Design review of the part built by this model. Coordinates are the model's own, in mm. A direction names the side the tool comes from. Coordinates: 2 decimals unless noted, no trailing zeros. Loops run counter-clockwise (first coordinate to the right, second up) from the corner with the lowest first, then second, coordinate; pieces in that order, holes last. Notation, with made-up numbers: (88.5, 64.5) -> (146.5, 64.5) arc R16 cw to (146.5, 95.5) -> close; hole circle Ø5 at (69, -28). An arc over 180 degrees is marked (long way). Answer as a JSON object with one key per item and string values.
```python
from build123d import *
from OCP.BRepFilletAPI import BRepFilletAPI_MakeChamfer

# Parameters (mm, degrees)
SKETCH_1_W          = 50
SKETCH_1_H          = 50
EXTRUDE_1_DEPTH     = 5
SKETCH_5_R          = 8
EXTRUDE_3_DEPTH     = 30
SKETCH_6_R          = 5.4
CUT_EXTRUDE_2_DEPTH = 50.749371855
FILLET_3_R          = 2
FILLET_2_SIZE       = 15
FILLET_2_SIZE_2     = 10
CHAMFER_1_SIZE      = 6
CHAMFER_1_SIZE2     = 2.797845949


with BuildPart() as part:
    # Эскиз1 → Бобышка-Вытянуть1 (new body)
    with BuildSketch(Plane(origin=(0, 0, 0), x_dir=(1, 0, 0), z_dir=(0, 1, 0))):
        Rectangle(SKETCH_1_W, SKETCH_1_H)
    extrude(amount=EXTRUDE_1_DEPTH)

    # Эскиз5 → Бобышка-Вытянуть3 (add)
    with BuildSketch(Plane(origin=(0, 5, 0), x_dir=(1, 0, 0), z_dir=(0, 1, 0))):
        with Locations(Location((0, 0, 0), (0, 0, 270))):
            Circle(SKETCH_5_R)
    extrude(amount=EXTRUDE_3_DEPTH)

    # Эскиз6 → Вырез-Вытянуть2 (cut, through all)
    with BuildSketch(Plane(origin=(0, 35, 0), x_dir=(1, 0, 0), z_dir=(0, 1, 0))):
        with Locations(Location((0, 0, 0), (0, 0, 270))):
            Circle(SKETCH_6_R)
    extrude(amount=-CUT_EXTRUDE_2_DEPTH, mode=Mode.SUBTRACT)

    # Скругление3
    fillet_3_edges = [part.edges().sort_by_distance(p)[0] for p in [
        (0, 35, -5.4),
    ]]
    fillet(fillet_3_edges, radius=FILLET_3_R)

    # Скругление2
    # an asymmetric fillet: 15, 10 mm, written as the material it adds along each edge
    with BuildSketch(Plane(origin=(0, 5, 0), x_dir=(0, 0, 1), z_dir=(-1, 0, 0))) as fillet_2_piece_1:
        with BuildLine():
            Bezier((8, FILLET_2_SIZE), (8, 0), (8 + FILLET_2_SIZE_2, 0), weights=[1, 0.707106781, 1])
            Line((8 + FILLET_2_SIZE_2, 0), (8, 0))
            Line((8, 0), (8, FILLET_2_SIZE))
        make_face()
    revolve(axis=Axis((0, 5, 0), (0, 1, 0)))

    # Фаска1: one chamfer whose edges measure the first distance from different faces: ONE call of the kernel's chamfer builder (chamfer() names one face for all edges)
    chamfer_1_edges_1 = [part.edges().sort_by_distance(p)[0] for p in [
        (0, 0, -5.4),
    ]]
    chamfer_1_side_1 = [part.faces().sort_by_distance(p)[0] for p in [
        (0, 16.5, -5.4),
    ]]
    chamfer_1_edges_2 = [part.edges().sort_by_distance(p)[0] for p in [
        (0, 0, 25),
        (-25, 0, 0),
        (0, 0, -25),
        (25, 0, 0),
    ]]
    chamfer_1_side_2 = [part.faces().sort_by_distance(p)[0] for p in [
        (0, 0, 24.292893219),
    ]]
    chamfer_1 = BRepFilletAPI_MakeChamfer(part.part.solid().wrapped)
    for e in chamfer_1_edges_1:
        chamfer_1.Add(CHAMFER_1_SIZE, CHAMFER_1_SIZE2, e.wrapped, chamfer_1_side_1[0].wrapped)  # the first distance lies on this face
    for e in chamfer_1_edges_2:
        chamfer_1.Add(CHAMFER_1_SIZE, CHAMFER_1_SIZE2, e.wrapped, chamfer_1_side_2[0].wrapped)  # the first distance lies on this face
    add(Compound.cast(chamfer_1.Shape()), mode=Mode.REPLACE)


solid = part.part
```
1) The part is to be moulded in two halves that separate along X. For faces 1 (the flat face through (-0.3, 1.4, 22)), 2 (the cylindrical face through (1.62, 19.69, 5.15)), 3 (the flat face through (25, 4, 0)), 4 (the flat face through (-22, 1.4, 0.3)), say which applies: pulls with the +X half, pulls with the -X half, needs draft (parallel to the pull), parting line crosses it, or undercut.
Completed:
{"face 1": "needs draft", "face 2": "undercut", "face 3": "pulls with the +X half", "face 4": "pulls with the -X half"}
2) For faces 5 (the flat face through (0, 4, 25)), 6 (the flat face through (-11, 5, -17)), list the 3-axis set-ups (+Z, -Z, +X, -X, +Y, -Y) from which the entire face can be reached by the end or side of a thin tool; tool diameter is ignored.
Completed:
{"face 5": "+Z, +X, -X, +Y, -Y", "face 6": "+Y"}
3) Add section A-A, the plane y = 22. Give the boundary of the cut face in (x, z), and give its area (3 significant figures).
Completed:
{"outline": "circle Ø16 at (0, 0); hole circle Ø10.8 at (0, 0)", "area": "109 mm²"}
4) Clearance check with flat-ended pins moving along their axes: pin 1 Ø3 at (y, z) = (19, -6) entering from -X; pin 2 Ø9.5 at (x, z) = (0, 0) entering from -Y; pin 3 Ø12 at (x, y) = (1, 22) entering from -Z. State where each tip first meets the part, or that it passes through.
Completed:
{"pin 1": "x = -6.64", "pin 2": "through", "pin 3": "z = -8.35"}
5) Add section B-B, the plane y = 3.5. Give the boundary of the cut face in (x, z), and give its area (3 significant figures).
Completed:
{"outline": "(-25, -25) -> (25, -25) -> (25, 25) -> (-25, 25) -> close; hole circle Ø13.13 at (0, 0)", "area": "2,360 mm²"}
6) Wall thickness on probe 1 along X at (y, z) = (19, 0); probe 2 along Z at (x, y) = (4.5, 10); probe 3 along Y at (x, z) = (19, 2.5): over which ranges is each line inside the solid? List them lowest first.
Completed:
{"probe 1": "-8.02 to -5.4, 5.4 to 8.02", "probe 2": "-9.54 to -2.98, 2.98 to 9.54", "probe 3": "0 to 5"}
